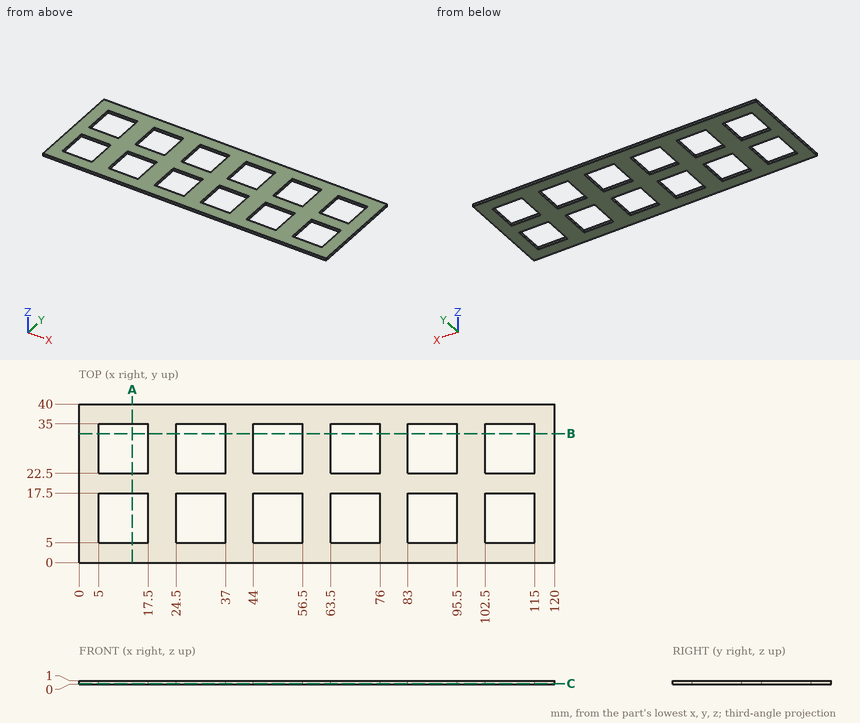
Job drawing, mm, ordinate dimensions from the low corner. One solid piece. Give positions to 0.01 mm unless a question says otherwise; leave off trailing zeros. Order: outer loops, then holes, each group sorted by start corner. A loop starts at its lowest first (then second) coordinate and runs counter-clockwise, first axis right, second up. Notation, with made-up numbers: M -31.75,-17 L -1.75,-17 A21 ccw -1.75,4 Z; hole C 73.25,12 d7. An arc over 180 degrees is marked long. Return JSON: item names as keys, results as strings.
Q1. Band-saw the part on A-A (x = 13.5). Give the cut face in (y, z).
Answer list:
{"outline": "M 0,0 L 5,0 L 5,1 L 0,1 Z; M 17.5,0 L 22.5,0 L 22.5,1 L 17.5,1 Z; M 35,0 L 40,0 L 40,1 L 35,1 Z"}
Q2. Band-saw the part on C-C (z = 0.2). Count the separate pieces of the cut face and the enclosed holes in it, then the cut area to 4 significant figures.
Answer list:
{"separate pieces": "1", "enclosed holes": "12", "area": "2,925 mm^2"}
Q3. Wall check: probe 1 along Y at (x, z) = (107, 0.15). Give the ranges that are in metal, low to high. Write a range as from..to.
Answer list:
{"probe 1": "y = 0..5, 17.5..22.5, 35..40"}
Q4. Band-saw the part on B-B (y = 32.5). Give the cut face in (x, z), then the cut area to 3 significant figures.
Answer list:
{"outline": "M 0,0 L 5,0 L 5,1 L 0,1 Z; M 17.5,0 L 24.5,0 L 24.5,1 L 17.5,1 Z; M 37,0 L 44,0 L 44,1 L 37,1 Z; M 56.5,0 L 63.5,0 L 63.5,1 L 56.5,1 Z; M 76,0 L 83,0 L 83,1 L 76,1 Z; M 95.5,0 L 102.5,0 L 102.5,1 L 95.5,1 Z; M 115,0 L 120,0 L 120,1 L 115,1 Z", "area": "45.0 mm^2"}
